Design review of the part built by this model. Coordinates are the model's own, in mm. Face numbers are marked on the shaded views. Round coordinates to 2 decimals unless told otherwise and drop trailing zeros. Loops run counter-clockwise (first coordinate to the right, second up) from the corner with the lowest first, then second, coordinate; pieces in that order, holes last. Notation, with made-up numbers: (80, 6) - (120, 6) arc R29 cw to (120, 32) - close; hole circle Ø6 at (40.5, 56.25). An arc over 180 degrees is marked (long way). Return JSON: item names as keys, results as strings. Group by question number.
(1) We need section C-C, the plane y = -5.25. Write out the cut boundary in (x, z).
(2) We need section A-A, the plane z = -0.25. Write out the cut boundary in (x, y), and give its area (3 significant figures).
(3) We need section D-D, the plane z = 1.5. Write out the cut boundary in (x, y).
(4) We need section B-B, the plane y = 8.5. Write out the cut boundary in (x, z).
(5) Wall thickness on L1, parallel to Y at x = 0, z = 0.3; L2, parallel to Y at x = 0.5, z = -1.25; L3, parallel to Z at x = -4.5, y = -5.25: over which ranges is each line inside the solid? List them lowest first. Write a range as [from, to].
(6) The part is to be moulded in two halves that separate along Y. For the marked faces 1, 2, 3 and 4, say which applies: pulls with the +Y half, pulls with the -Y half, needs draft (parallel to the pull), parting line crosses it, or undercut.
(7) Clearance check with flat-ended pins moving along their axes: pin 1 (0.5 mm diameter, centred on y = -5.5, z = -3, fed in from -X); pin 2 (4 mm diameter, centred on x = 0.5, y = -2.5, fed in from -Z); pin 3 (3 mm diameter, centred on y = -7, z = -1, fed in from +X). State where each tip first meets the part, or that it passes through.
Solid Edge part; units mm, degrees
sketch "Sketch1" plane through (0, 0, 0) normal (0, 0, 1) x (1, 0, 0)
  circle A0 centre (0, 0) radius 10
  circle A1 centre (0, 8.5) radius 0.75
  circle A2 centre (0, -8.5) radius 0.75
extrude "Protrusion1" add sketch "Sketch1" along normal blind 1
sketch "Sketch2" plane through (0, 0, 0) normal (0, 0, -1) x (1, 0, 0)
  line L0 (-2.5, 5) -> (2.5, 5)
  line L1 (2.5, 5) -> (2.5, 6)
  line L2 (2.5, 6) -> (-2.5, 6)
  line L3 (-2.5, 6) -> (-2.5, 5)
  line L4 (-2.5, -5) -> (2.5, -5)
  line L5 (2.5, -5) -> (2.5, -6)
  line L6 (2.5, -6) -> (-2.5, -6)
  line L7 (-2.5, -6) -> (-2.5, -5)
extrude "ExtrudedProtrusion_3" add sketch "Sketch2" along normal blind 5
sketch "Sketch3" plane through (0, 0, 1) normal (0, 0, 1) x (0, -1, 0)
  circle A0 centre (0, 0) radius 1.5
extrude "ExtrudedProtrusion_4" add sketch "Sketch3" along normal blind 1
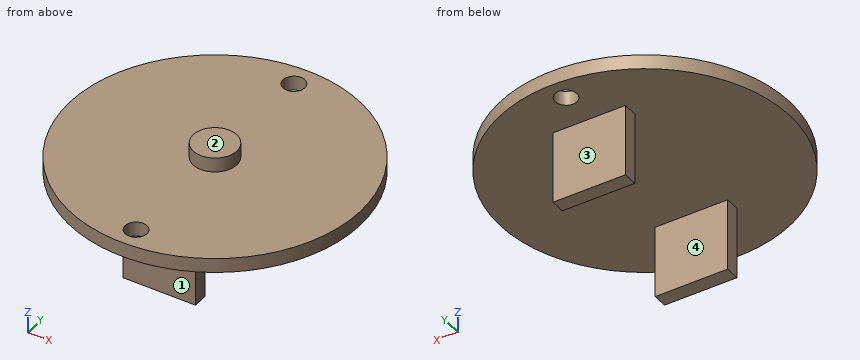
Solutions:
{
 "1": {"outline": "(-8.51, 0) - (-2.5, 0) - (-2.5, -5) - (2.5, -5) - (2.5, 0) - (8.51, 0) - (8.51, 1) - (-8.51, 1) - close"},
 "2": {"outline": "(-2.5, -6) - (2.5, -6) - (2.5, -5) - (-2.5, -5) - close; (-2.5, 5) - (2.5, 5) - (2.5, 6) - (-2.5, 6) - close", "area": "10.0 mm^2"},
 "3": {"outline": "circle Ø3 at (0, 0)"},
 "4": {"outline": "(-5.27, 0) - (-0.75, 0) - (-0.75, 1) - (-5.27, 1) - close; (0.75, 0) - (5.27, 0) - (5.27, 1) - (0.75, 1) - close"},
 "5": {"L1": "[-10, -9.25], [-7.75, 7.75], [9.25, 10]", "L2": "[-6, -5], [5, 6]", "L3": "[0, 1]"},
 "6": {"face 1": "pulls with the -Y half", "face 2": "needs draft", "face 3": "pulls with the +Y half", "face 4": "undercut"},
 "7": {"pin 1": "x = -2.5", "pin 2": "z = 0", "pin 3": "x = 8.09"}
}
